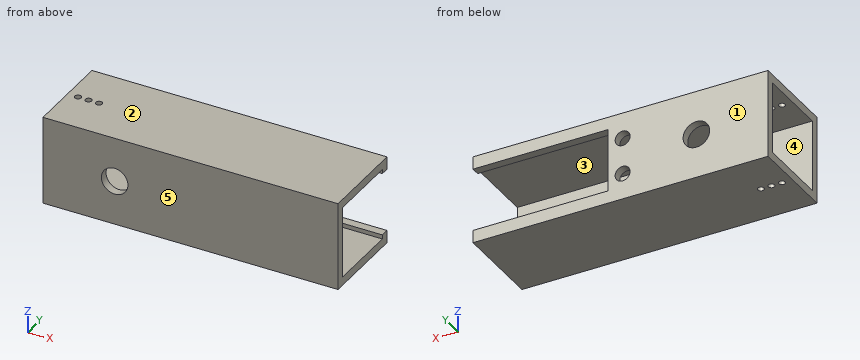
from build123d import *

# Parameters (mm, degrees)
SKETCH1_W           = 26.67
SKETCH1_H           = 26.67
SKETCH1_W_2         = 21.59
SKETCH1_H_2         = 21.59
BOSS_EXTRUDE1_DEPTH = 88.9
SKETCH2_R           = 4.0005
CUT_EXTRUDE1_DEPTH  = 94.767377723
CUT_EXTRUDE2_REACH  = 95.767
SKETCH3_R           = 2.25
SKETCH3_W           = 40.64
SKETCH3_H           = 19.05
SKETCH4_R           = 0.9525
CUT_EXTRUDE3_DEPTH  = 94.767377723


with BuildPart() as part:
    # Sketch1 → Boss-Extrude1 (new body)
    with BuildSketch(Plane(origin=(0, 0, 0), x_dir=(0, 0, -1), z_dir=(1, 0, 0))):
        Rectangle(SKETCH1_W, SKETCH1_H)
        Rectangle(SKETCH1_W_2, SKETCH1_H_2, mode=Mode.SUBTRACT)
    extrude(amount=BOSS_EXTRUDE1_DEPTH)

    # Sketch2 → Cut-Extrude1 (cut, through all)
    with BuildSketch(Plane(origin=(0, 13.335, 0), x_dir=(1, 0, 0), z_dir=(0, 1, 0))):
        with Locations(Location((21.59, 0, 0), (0, 0, 270))):
            Circle(SKETCH2_R)
    extrude(amount=-CUT_EXTRUDE1_DEPTH, mode=Mode.SUBTRACT)

    # Sketch3 → Cut-Extrude2 (cut, up to next)
    with BuildSketch(Plane(origin=(0, 13.335, 0), x_dir=(1, 0, 0), z_dir=(0, 1, 0)), mode=Mode.PRIVATE) as cut_extrude2_sk1:
        with Locations(Location((43.815, 5.487743894, 0), (0, 0, 270))):
            Circle(SKETCH3_R)
    cut_extrude2_tool1 = extrude(cut_extrude2_sk1.sketch, amount=-CUT_EXTRUDE2_REACH, mode=Mode.PRIVATE) & part.part
    # Sketch3 → Cut-Extrude2 (cut, up to next)
    with BuildSketch(Plane(origin=(0, 13.335, 0), x_dir=(1, 0, 0), z_dir=(0, 1, 0)), mode=Mode.PRIVATE) as cut_extrude2_sk2:
        with Locations(Location((43.815, -5.487743894, 0), (0, 0, 270))):
            Circle(SKETCH3_R)
    cut_extrude2_tool2 = extrude(cut_extrude2_sk2.sketch, amount=-CUT_EXTRUDE2_REACH, mode=Mode.PRIVATE) & part.part
    # Sketch3 → Cut-Extrude2 (cut, up to next)
    with BuildSketch(Plane(origin=(0, 13.335, 0), x_dir=(1, 0, 0), z_dir=(0, 1, 0)), mode=Mode.PRIVATE) as cut_extrude2_sk3:
        with Locations((68.58, 0)):
            Rectangle(SKETCH3_W, SKETCH3_H)
    cut_extrude2_tool3 = extrude(cut_extrude2_sk3.sketch, amount=-CUT_EXTRUDE2_REACH, mode=Mode.PRIVATE) & part.part
    add(cut_extrude2_tool1.solids().sort_by_distance((43.815, 13.335, -5.487744))[0], mode=Mode.SUBTRACT)
    add(cut_extrude2_tool2.solids().sort_by_distance((43.815, 13.335, 5.487744))[0], mode=Mode.SUBTRACT)
    add(cut_extrude2_tool3.solids().sort_by_distance((68.58, 13.335, 0))[0], mode=Mode.SUBTRACT)

    # Sketch4 → Cut-Extrude3 (cut, through all)
    with BuildSketch(Plane.XY.offset(13.335)):
        with Locations((6.35, 0)):
            Circle(SKETCH4_R)
        with Locations((3.175, 0)):
            Circle(SKETCH4_R)
        with Locations((9.525, 0)):
            Circle(SKETCH4_R)
    extrude(amount=-CUT_EXTRUDE3_DEPTH, mode=Mode.SUBTRACT)


solid = part.part
Could you check a few things on this model? Use its own coordinates, in mm. Face numbers are marked on the shaded views. A direction names the side the tool comes from. Give positions to 0.01 mm unless a question says otherwise; leave off trailing zeros. Order: outer loops, then holes, each group sorted by start corner. A loop starts at its lowest first (then second) coordinate and runs counter-clockwise, first axis right, second up.
1. Suppose I cut it at B-B (z = 0). List the corners of the cut face in (x, y) for me (1 decimal), plus the area to 3 significant figures.
2. Suppose I cut it at D-D (y = 5.25). List the corners of the cut face in (x, z) for me (3 decimals).
3. Suppose I cut it at A-A (x = 21.59). List the corners of the cut face in (y, z) for me (1 decimal).
4. We'd pull the mould along Y, two halves only. Please class the marked faces 1, 2 and 3: pulls with the +Y half, pulls with the -Y half, needs draft (parallel to the pull), parting line crosses it, or undercut.
5. For the marked faces 4 and 5, which set-ups out of +Z, -Z, +X, -X, +Y, -Y let a thin tool reach every point of the face, with its end or its side?
6. Suppose I cut it at C-C (y = 0). Give the number of separate pieces and of enclosed holes in the cut face, plus the area to 3 significant figures.
7. I need wall thicknesses on L1, parallel to Y at x = 9.5, z = -8.75 (3 decimals); L2, parallel to X at y = 12.45, z = 0. Which ranges of each line are inside material? Lowest first, please.
8. Will these pins go through, and if not, where does the flat tip stop? P1, Ø8, axis at y = 10, z = -3, coming from the +X side; P2, Ø2, axis at x = 3.175, y = 0, coming from the -Z side (3 decimals); P3, Ø4, axis at x = 43.82, z = -5.49, coming from the +Y side (3 decimals).
Solved:
1. outline: (0, -13.3) - (17.6, -13.3) - (17.6, -10.8) - (0, -10.8) - close; (0, 10.8) - (17.6, 10.8) - (17.6, 13.3) - (0, 13.3) - close; (25.6, -13.3) - (88.9, -13.3) - (88.9, -10.8) - (25.6, -10.8) - close; (25.6, 10.8) - (48.3, 10.8) - (48.3, 13.3) - (25.6, 13.3) - close
1. area: 308 mm2
2. outline: (0, -13.335) - (88.9, -13.335) - (88.9, -10.795) - (0, -10.795) - close; (0, 10.795) - (88.9, 10.795) - (88.9, 13.335) - (0, 13.335) - close
3. outline: (-13.3, -13.3) - (13.3, -13.3) - (13.3, -4) - (10.8, -4) - (10.8, -10.8) - (-10.8, -10.8) - (-10.8, -4) - (-13.3, -4) - close; (-13.3, 4) - (-10.8, 4) - (-10.8, 10.8) - (10.8, 10.8) - (10.8, 4) - (13.3, 4) - (13.3, 13.3) - (-13.3, 13.3) - close
4. face 1: pulls with the +Y half
4. face 2: needs draft
4. face 3: undercut
5. face 4: +X, -X
5. face 5: +Z, -Z, +X, -X, -Y
6. separate pieces: 8
6. enclosed holes: 0
6. area: 423 mm2
7. L1: y = -13.335 to -10.795, 10.795 to 13.335
7. L2: x = 0 to 17.59, 25.59 to 48.26
8. P1: stops at x = 48.26
8. P2: stops at z = -13.335
8. P3: stops at y = -10.795
